```python
from build123d import *

# Parameters (mm, degrees)
SKETCH_W     = 72
SKETCH_H     = 95
PAD_DEPTH    = 1.6
SKETCH001_R  = 1.6
POCKET_DEPTH = 1.601
SKETCH006_W  = 45
SKETCH006_H  = 29
PAD004_DEPTH = 12
SKETCH005_W  = 52
SKETCH005_H  = 29
PAD005_DEPTH = 1.6
SKETCH011_W  = 8
SKETCH011_H  = 8
PAD008_DEPTH = 3
SKETCH013_W  = 56
SKETCH013_H  = 1.5
PAD010_DEPTH = 10
SKETCH014_W  = 50
SKETCH014_H  = 25
PAD011_DEPTH = 5.5


with BuildPart() as part:
    # Sketch → Pad (new body)
    with BuildSketch(Plane.XY):
        with Locations((36, 47.5)):
            Rectangle(SKETCH_W, SKETCH_H)
    extrude(amount=PAD_DEPTH)

    # Sketch001 (on Face6 of Pad) → Pocket (cut, through all)
    with BuildSketch(Plane.XY.offset(1.6)):
        with Locations((3, 3)):
            Circle(SKETCH001_R)
        with Locations((69, 3)):
            Circle(SKETCH001_R)
        with Locations((69, 92)):
            Circle(SKETCH001_R)
        with Locations((3, 92)):
            Circle(SKETCH001_R)
    extrude(amount=-POCKET_DEPTH, mode=Mode.SUBTRACT)

    # Sketch006 (on Face5 of Pocket) → Pad004 (join)
    with BuildSketch(Plane.XY.offset(1.6)):
        with Locations((49.5, 20.5)):
            Rectangle(SKETCH006_W, SKETCH006_H)
    extrude(amount=PAD004_DEPTH)

    # Sketch005 (on Face5 of Pocket) → Pad005 (join)
    with BuildSketch(Plane.XY.offset(13.6)):
        with Locations((53, 20.5)):
            Rectangle(SKETCH005_W, SKETCH005_H)
    extrude(amount=PAD005_DEPTH)

    # Sketch011 (on Face20 of Pad005) → Pad008 (join)
    with BuildSketch(Plane.XY.offset(15.2)):
        with Locations((75, 20.5)):
            Rectangle(SKETCH011_W, SKETCH011_H)
    extrude(amount=PAD008_DEPTH)

    # Sketch013 (on Face5 of Pad008) → Pad010 (join)
    with BuildSketch(Plane.XY.offset(1.6)):
        with Locations((36, 89.75)):
            Rectangle(SKETCH013_W, SKETCH013_H)
    extrude(amount=PAD010_DEPTH)

    # Sketch014 (on Face5 of Pad010) → Pad011 (join)
    with BuildSketch(Plane.XY.offset(1.6)):
        with Locations((35, 67.5)):
            Rectangle(SKETCH014_W, SKETCH014_H)
    extrude(amount=PAD011_DEPTH)


solid = part.part
```
Geometry: final body of the model. Coordinates: model frame, mm. A direction names the side the tool comes from. Coordinates: 2 decimals unless noted, no trailing zeros. Order: outer loops, then holes, each group sorted by start corner. A loop starts at its lowest first (then second) coordinate and runs counter-clockwise, first axis right, second up. Notation, with made-up numbers: (66.25, 30) -> (80.25, 30) arc R20 ccw to (80.25, 60) -> close; hole circle Ø1 at (78.5, -24). An arc over 180 degrees is marked (long way). Answer in a Markdown table with one row per item.
Item 1: Contact query for flat-ended pins moving along their axis: P1, Ø1.6, axis at x = 43.5, z = 3.5, coming from the +Y side; P2, Ø6, axis at x = 46.5, y = 66.5, coming from the -Z side; P3, Ø1.5, axis at x = 74.5, z = 16, coming from the +Y side; P4, Ø4, axis at x = 69, y = 92, coming from the +Z side. Output: stop coordinate, or through.
Return value:
| item | result |
|---|---|
| P1 | stops at y = 90.5 |
| P2 | stops at z = 0 |
| P3 | stops at y = 24.5 |
| P4 | stops at z = 1.6 |
Item 2: Draft query along Y for faces 1 (the flat face through (35, 48, 0)), 2 (the flat face through (35, 38, 1.6)), 3 (the flat face through (75, 24.5, 17)). Return one class per face: released by +Y, released by -Y, zero draft, split by the parting line, or undercut.
Return value:
| item | result |
|---|---|
| face 1 | zero draft |
| face 2 | undercut |
| face 3 | released by +Y |
Item 3: Section D-D on z = 3. Output: boundary loops of the cut face in (x, y), plus the area to 3 significant figures.
Return value:
| item | result |
|---|---|
| outline | (8, 89) -> (64, 89) -> (64, 90.5) -> (8, 90.5) -> close; (10, 55) -> (60, 55) -> (60, 80) -> (10, 80) -> close; (27, 6) -> (72, 6) -> (72, 35) -> (27, 35) -> close |
| area | 2,640 mm² |
Item 4: Section B-B on z = 10.5. Output: boundary loops of the cut face in (x, y), plus the area to 3 significant figures.
Return value:
| item | result |
|---|---|
| outline | (8, 89) -> (64, 89) -> (64, 90.5) -> (8, 90.5) -> close; (27, 6) -> (72, 6) -> (72, 35) -> (27, 35) -> close |
| area | 1,390 mm² |
Item 5: Access query for faces 4 (the flat face through (75, 16.5, 17)), 5 (the flat face through (36, 89, 7)), 6 (the flat face through (27, 20, 8)). Directions: +Z, -Z, +X, -X, +Y, -Y. A direction counts if a zero-diameter tool reaches every point of the face in a straight line with its end or side. Return the directions, or none.
Return value:
| item | result |
|---|---|
| face 4 | +Z, +X, -X, -Y |
| face 5 | +Z, +X, -X |
| face 6 | +Z, -X, -Y |
Item 6: Section A-A on x = 69. Output: boundary loops of the cut face in (y, z), plus the area to 3 significant figures.
Return value:
| item | result |
|---|---|
| outline | (0, 0) -> (1.4, 0) -> (1.4, 1.6) -> (0, 1.6) -> close; (4.6, 0) -> (90.4, 0) -> (90.4, 1.6) -> (35, 1.6) -> (35, 15.2) -> (6, 15.2) -> (6, 1.6) -> (4.6, 1.6) -> close; (93.6, 0) -> (95, 0) -> (95, 1.6) -> (93.6, 1.6) -> close |
| area | 536 mm² |
Item 7: Ray query, L1, parallel to X at y = 92, z = 0.55; L2, parallel to Y at x = 3, z = 1; L3, parallel to Y at x = 45, z = 4.75. Return the intervals inside material, ascending.
Return value:
| item | result |
|---|---|
| L1 | x = 0 to 1.4, 4.6 to 67.4, 70.6 to 72 |
| L2 | y = 0 to 1.4, 4.6 to 90.4, 93.6 to 95 |
| L3 | y = 6 to 35, 55 to 80, 89 to 90.5 |
Item 8: Section C-C on y = 3. Output: boundary loops of the cut face in (x, z).
Return value:
| item | result |
|---|---|
| outline | (0, 0) -> (1.4, 0) -> (1.4, 1.6) -> (0, 1.6) -> close; (4.6, 0) -> (67.4, 0) -> (67.4, 1.6) -> (4.6, 1.6) -> close; (70.6, 0) -> (72, 0) -> (72, 1.6) -> (70.6, 1.6) -> close |
